Read the model definition and answer for the solid it produces. Units are mm, in the model's axes. Face numbers are marked on the shaded views. A direction names the side the tool comes from. Coordinates: 2 decimals unless noted, no trailing zeros. Order: outer loops, then holes, each group sorted by start corner. A loop starts at its lowest first (then second) coordinate and runs counter-clockwise, first axis right, second up. Notation, with made-up numbers: (-36.5, -25) - (-5.5, -25) arc R29 ccw to (-5.5, -5) - close; hole circle Ø8 at (8, 62). An arc over 180 degrees is marked (long way). Answer as a JSON object with one key per item and string values. Group by question number.
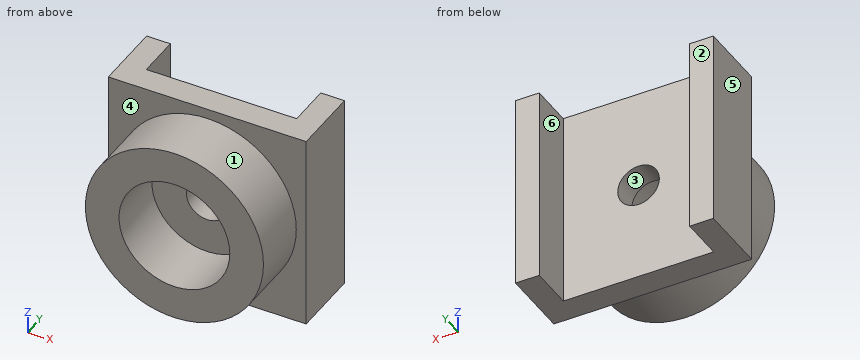
from build123d import *

# Parameters (mm, degrees)
ESBO_O1_R                = 4.5
RESSALTO_EXTRUS_O1_DEPTH = 3
ESBO_O2_R                = 2.8
CORTE_EXTRUS_O1_DEPTH    = 4
ESBO_O3_W                = 10
ESBO_O3_H                = 10
RESSALTO_EXTRUS_O2_DEPTH = 3.5
ESBO_O4_W                = 7.6
ESBO_O4_H                = 10
CORTE_EXTRUS_O2_DEPTH    = 2.2
ESBO_O5_R                = 1.050702539
CORTE_EXTRUS_O3_DEPTH    = 5.3


with BuildPart() as part:
    # Esboço1 → Ressalto-extrusão1 (new body)
    with BuildSketch(Plane(origin=(0, 0, 0), x_dir=(1, 0, 0), z_dir=(0, 1, 0))):
        Circle(ESBO_O1_R)
    extrude(amount=RESSALTO_EXTRUS_O1_DEPTH)

    # Esboço2 → Corte-extrusão1 (cut, through all)
    with BuildSketch(Plane(origin=(0, 3, 0), x_dir=(1, 0, 0), z_dir=(0, 1, 0))):
        Circle(ESBO_O2_R)
    extrude(amount=-CORTE_EXTRUS_O1_DEPTH, mode=Mode.SUBTRACT)

    # Esboço3 → Ressalto-extrusão2 (add)
    with BuildSketch(Plane(origin=(0, 3, 0), x_dir=(1, 0, 0), z_dir=(0, 1, 0))):
        Rectangle(ESBO_O3_W, ESBO_O3_H)
    extrude(amount=RESSALTO_EXTRUS_O2_DEPTH)

    # Esboço4 → Corte-extrusão2 (cut)
    with BuildSketch(Plane(origin=(0, 6.5, 0), x_dir=(1, 0, 0), z_dir=(0, 1, 0))):
        Rectangle(ESBO_O4_W, ESBO_O4_H)
    extrude(amount=-CORTE_EXTRUS_O2_DEPTH, mode=Mode.SUBTRACT)

    # Esboço5 → Corte-extrusão3 (cut, through all)
    with BuildSketch(Plane(origin=(0, 4.3, 0), x_dir=(1, 0, 0), z_dir=(0, 1, 0))):
        Circle(ESBO_O5_R)
    extrude(amount=-CORTE_EXTRUS_O3_DEPTH, mode=Mode.SUBTRACT)


solid = part.part
1. A cutting plane is placed at B-B on y = 5. Write down the section's boundary in (x, z).
2. Straight lines are drawn through the part: L1, parallel to X at y = 1.8, z = 0; L2, parallel to X at y = 3.45, z = 0. For each, find the intervals that lie inside material, in ascending order.
3. For the marked faces 4, 5 and 6, determine the directions among +Z, -Z, +X, -X, +Y, -Y from which every point of the face is accessible in a straight line to the end or side of a thin tool.
4. A cutting plane is placed at A-A on z = 0. Write down the section's boundary in (x, y), and give its area (3 significant figures).
5. A cutting plane is placed at D-D on y = 3.75. Write down the section's boundary in (x, z), and give its area (3 significant figures).
6. Given pin 1 (2.5 mm diameter, centred on x = 0, z = 0, fed in from +Y), flat-ended and moving along its own axis, determine where the tip first touches the part or whether it passes through.
7. For a pull along Z with two mould halves and no side action, classify the marked faces 1, 2 and 3 as pulls with the +Z half, pulls with the -Z half, needs draft (parallel to the pull), parting line crosses it, or undercut.
8. A cutting plane is placed at C-C on x = 0. Write down the section's boundary in (y, z), and give its area (3 significant figures).
Derived:
{
 "1": {"outline": "(-5, -5) - (-3.8, -5) - (-3.8, 5) - (-5, 5) - close; (3.8, -5) - (5, -5) - (5, 5) - (3.8, 5) - close"},
 "2": {"L1": "x = -4.5 to -2.8, 2.8 to 4.5", "L2": "x = -5 to -1.05, 1.05 to 5"},
 "3": {"face 4": "-Y", "face 5": "+Z, -Z, -X, +Y, -Y", "face 6": "+Z, -Z, +Y"},
 "4": {"outline": "(-5, 3) - (-4.5, 3) - (-4.5, 0) - (-2.8, 0) - (-2.8, 3) - (-1.05, 3) - (-1.05, 4.3) - (-3.8, 4.3) - (-3.8, 6.5) - (-5, 6.5) - close; (1.05, 3) - (2.8, 3) - (2.8, 0) - (4.5, 0) - (4.5, 3) - (5, 3) - (5, 6.5) - (3.8, 6.5) - (3.8, 4.3) - (1.05, 4.3) - close", "area": "25.7 mm2"},
 "5": {"outline": "(-5, -5) - (5, -5) - (5, 5) - (-5, 5) - close; hole circle Ø2.1 at (0, 0)", "area": "96.5 mm2"},
 "6": {"pin 1": "stops at y = 4.3"},
 "7": {"face 1": "parting line crosses it", "face 2": "needs draft", "face 3": "undercut"},
 "8": {"outline": "(0, -4.5) - (3, -4.5) - (3, -5) - (4.3, -5) - (4.3, -1.05) - (3, -1.05) - (3, -2.8) - (0, -2.8) - close; (0, 2.8) - (3, 2.8) - (3, 1.05) - (4.3, 1.05) - (4.3, 5) - (3, 5) - (3, 4.5) - (0, 4.5) - close", "area": "20.5 mm2"}
}
